Check sheet for the modelled part. Datum: model origin and axes. Units: mm. A direction names the side the tool comes from. Give positions to 0.01 mm unless a question says otherwise; leave off trailing zeros. Order: outer loops, then holes, each group sorted by start corner. A loop starts at its lowest first (then second) coordinate and runs counter-clockwise, first axis right, second up. Notation, with made-up numbers: (66.25, 82.5) -> (98.25, 82.5) arc R24 cw to (98.25, 107.5) -> close; hole circle Ø2 at (84.5, 12). An arc over 180 degrees is marked (long way). Answer in a Markdown table with one row per item. Add a question column.
(1) Go/stop test with flat-tipped pins: pin 1 (12 mm diameter, centred on y = -14.5, z = -11, fed in from +X); pin 2 (1 mm diameter, centred on y = -9.5, z = -28, fed in from +X); pin 3 (6 mm diameter, centred on x = -42, y = -17.5, fed in from +Z); pin 4 (4 mm diameter, centred on x = 17.5, z = 16, fed in from -Y). Record where each tip stops, or that it passes through.
(2) Thickness scan on L1, parallel to Z at x = -53, y = -6; L2, parallel to Z at x = -33, y = -16.5; L3, parallel to Z at x = -11, y = -12.25 (3 decimals). Record the ranges inside material, lowest first. Write a range as [from, to].
(3) Cross-section at B-B (y = -9.5). State how many separate pieces and enclosed holes the cut face has, then the cut area to 3 significant figures.
(4) Cross-section at A-A (x = 0). Record the cut outline in (y, z).
(5) Release check for a two-part mould opening along Z. For faces 6 (the face through (49.733, -9.86, 5.165)), 7 (the face through (-10.34, -9.86, 48.92)), 8 (the face through (31, 0, 36)) record: released by +Z, released by -Z, zero draft, split by the parting line, or undercut.
(6) Set-up check for faces 1 (the face through (-49.72, -9.86, 5.29)), 2 (the face through (5.832, -9.86, -54.889)), 3 (the face through (10.456, -9.86, 48.895)), 4 (the face through (-7.353, -9.86, -10.17)), 5 (the face through (45.01, -9.86, 40.43)): record each of +Z, -Z, +X, -X, +Y, -Y from which the full face is reachable in a straight line by a thin tool's end or side.
```python
from build123d import *

# Parameters (mm, degrees)
F1_R     = 50
F2_DEPTH = 20
F4_DEPTH = 20
F5_R     = 45
F5_R_2   = 16
F6_DEPTH = 8
F7_R     = 10
F8_DEPTH = 25
F9_SIZE  = 2
F10_R    = 3


with BuildPart() as f2:
    # F1 (on Front) → F2 (new body)
    with BuildSketch(Plane.XZ):
        Circle(F1_R)
        with BuildLine():
            ThreePointArc((-2.05, 12.3814377194), (0, 12.55), (2.05, 12.3814377194))
            Line((2.05, 12.3814377194), (2.05, 10.2979366865))
            ThreePointArc((2.05, 10.2979366865), (3.2446784409, 9.9860934211), (4.3944904749, 9.5361655536))
            Line((4.3944904749, 9.5361655536), (5.6191416552, 11.221753297))
            ThreePointArc((5.6191416552, 11.221753297), (7.3767049163, 10.1531632794), (8.9361113321, 8.8118337626))
            Line((8.9361113321, 8.8118337626), (7.7114601519, 7.1262460192))
            ThreePointArc((7.7114601519, 7.1262460192), (8.4946784409, 6.1717451491), (9.1604349517, 5.1319033015))
            Line((9.1604349517, 5.1319033015), (11.1419621857, 5.7757405285))
            ThreePointArc((11.1419621857, 5.7757405285), (11.9357592795, 3.8781632794), (12.4089318626, 1.8764088117))
            Line((12.4089318626, 1.8764088117), (10.4274046286, 1.2325715847))
            ThreePointArc((10.4274046286, 1.2325715847), (10.4818354452, 0.6173537882), (10.5, 0))
            ThreePointArc((10.5, 0), (10.4818354452, -0.6173537882), (10.4274046286, -1.2325715847))
            Line((10.4274046286, -1.2325715847), (12.4089318626, -1.8764088117))
            ThreePointArc((12.4089318626, -1.8764088117), (11.9357592795, -3.8781632794), (11.1419621857, -5.7757405285))
            Line((11.1419621857, -5.7757405285), (9.1604349517, -5.1319033015))
            ThreePointArc((9.1604349517, -5.1319033015), (8.4946784409, -6.1717451491), (7.7114601519, -7.1262460192))
            Line((7.7114601519, -7.1262460192), (8.9361113321, -8.8118337626))
            ThreePointArc((8.9361113321, -8.8118337626), (7.3767049163, -10.1531632794), (5.6191416552, -11.221753297))
            Line((5.6191416552, -11.221753297), (4.3944904749, -9.5361655536))
            ThreePointArc((4.3944904749, -9.5361655536), (3.2446784409, -9.9860934211), (2.05, -10.2979366865))
            Line((2.05, -10.2979366865), (2.05, -12.3814377194))
            ThreePointArc((2.05, -12.3814377194), (0, -12.55), (-2.05, -12.3814377194))
            Line((-2.05, -12.3814377194), (-2.05, -10.2979366865))
            ThreePointArc((-2.05, -10.2979366865), (-3.2446784409, -9.9860934211), (-4.3944904749, -9.5361655536))
            Line((-4.3944904749, -9.5361655536), (-5.6191416552, -11.221753297))
            ThreePointArc((-5.6191416552, -11.221753297), (-7.3767049163, -10.1531632794), (-8.9361113321, -8.8118337626))
            Line((-8.9361113321, -8.8118337626), (-7.7114601519, -7.1262460192))
            ThreePointArc((-7.7114601519, -7.1262460192), (-8.4946784409, -6.1717451491), (-9.1604349517, -5.1319033015))
            Line((-9.1604349517, -5.1319033015), (-11.1419621857, -5.7757405285))
            ThreePointArc((-11.1419621857, -5.7757405285), (-11.9357592795, -3.8781632794), (-12.4089318626, -1.8764088117))
            Line((-12.4089318626, -1.8764088117), (-10.4274046286, -1.2325715847))
            ThreePointArc((-10.4274046286, -1.2325715847), (-10.5, 0), (-10.4274046286, 1.2325715847))
            Line((-10.4274046286, 1.2325715847), (-12.4089318626, 1.8764088117))
            ThreePointArc((-12.4089318626, 1.8764088117), (-11.9357592795, 3.8781632794), (-11.1419621857, 5.7757405285))
            Line((-11.1419621857, 5.7757405285), (-9.1604349517, 5.1319033015))
            ThreePointArc((-9.1604349517, 5.1319033015), (-8.4946784409, 6.1717451491), (-7.7114601519, 7.1262460192))
            Line((-7.7114601519, 7.1262460192), (-8.9361113321, 8.8118337626))
            ThreePointArc((-8.9361113321, 8.8118337626), (-7.3767049163, 10.1531632794), (-5.6191416552, 11.221753297))
            Line((-5.6191416552, 11.221753297), (-4.3944904749, 9.5361655536))
            ThreePointArc((-4.3944904749, 9.5361655536), (-3.2446784409, 9.9860934211), (-2.05, 10.2979366865))
            Line((-2.05, 10.2979366865), (-2.05, 12.3814377194))
        make_face(mode=Mode.SUBTRACT)
    extrude(amount=F2_DEPTH)

    # F3 (on Front) → F4 (join)
    with BuildSketch(Plane.XZ):
        with BuildLine():
            ThreePointArc((6.0454455831, 49.6331803102), (5.6999328162, 54.9765582241), (5.0372687356, 60.2899321917))
            ThreePointArc((5.0372687356, 60.2899321917), (0, 60.5), (-5.0372687356, 60.2899321917))
            ThreePointArc((-5.0372687356, 60.2899321917), (-5.6999328162, 54.9765582241), (-6.0454455831, 49.6331803102))
            ThreePointArc((-6.0454455831, 49.6331803102), (0, 50), (6.0454455831, 49.6331803102))
        make_face()
        with BuildLine():
            ThreePointArc((19.9203506586, 57.1264354711), (17.1538330068, 52.5419565819), (14.6648437927, 47.8010706631))
            ThreePointArc((14.6648437927, 47.8010706631), (20.3368321538, 45.6772728821), (25.7104224964, 42.8832621783))
            ThreePointArc((25.7104224964, 42.8832621783), (27.5681284731, 47.905213503), (29.1238986033, 53.0287519196))
            ThreePointArc((29.1238986033, 53.0287519196), (24.6075669061, 55.2695001874), (19.9203506586, 57.1264354711))
        make_face()
        with BuildLine():
            ThreePointArc((41.4335604532, 44.0852590802), (37.0415452653, 41.022373318), (32.8394484508, 37.7037216393))
            ThreePointArc((32.8394484508, 37.7037216393), (37.1572412739, 33.4565303179), (40.9298337882, 28.7184384337))
            ThreePointArc((40.9298337882, 28.7184384337), (44.6695442683, 32.5506221621), (48.1747418201, 36.5984186894))
            ThreePointArc((48.1747418201, 36.5984186894), (44.9602619414, 40.4824016847), (41.4335604532, 44.0852590802))
        make_face()
        with BuildLine():
            ThreePointArc((55.7825312334, 23.4213408923), (50.5244378355, 22.4096490308), (45.3358141347, 21.0870566164))
            ThreePointArc((45.3358141347, 21.0870566164), (47.5528258148, 15.4508497187), (49.0721049822, 9.587935785))
            ThreePointArc((49.0721049822, 9.587935785), (54.0471900496, 11.5677325362), (58.8957345225, 13.8398863816))
            ThreePointArc((58.8957345225, 13.8398863816), (57.5389192359, 18.6955281597), (55.7825312334, 23.4213408923))
        make_face()
        with BuildLine():
            ThreePointArc((60.486195595, -1.2923399121), (55.2711961039, -0.077907159), (49.9932056918, 0.8242479348))
            ThreePointArc((49.9932056918, 0.8242479348), (49.9983013941, 0.4121379686), (50, 0))
            ThreePointArc((50, 0), (49.6813253191, -5.6361258444), (48.7293634187, -11.2004080646))
            ThreePointArc((48.7293634187, -11.2004080646), (54.0795856679, -11.4153231348), (59.433119675, -11.3116880129))
            ThreePointArc((59.433119675, -11.3116880129), (60.1685746698, -6.3239720277), (60.486195595, -1.2923399121))
        make_face()
        with BuildLine():
            ThreePointArc((54.7312472383, -25.7825634052), (50.4610624428, -22.5519924933), (46.0063178108, -19.5810807029))
            ThreePointArc((46.0063178108, -19.5810807029), (43.3012701892, -25), (39.9608722277, -30.0520996073))
            ThreePointArc((39.9608722277, -30.0520996073), (44.7611296266, -32.4245657308), (49.6939785027, -34.5073687866))
            ThreePointArc((49.6939785027, -34.5073687866), (52.394536929, -30.25), (54.7312472383, -25.7825634052))
        make_face()
        with BuildLine():
            ThreePointArc((39.5127690163, -45.8147474582), (36.9257526611, -41.1266334471), (34.064519626, -36.6006625985))
            ThreePointArc((34.064519626, -36.6006625985), (29.3892626146, -40.4508497187), (24.2827831954, -43.7075101131))
            ThreePointArc((24.2827831954, -43.7075101131), (27.7030676308, -47.827306344), (31.3622969917, -51.7364120075))
            ThreePointArc((31.3622969917, -51.7364120075), (35.5610077637, -48.9455281597), (39.5127690164, -45.8147474582))
        make_face()
        with BuildLine():
            ThreePointArc((17.4621740692, -57.9251454618), (17.0056447843, -52.5901058542), (16.2326565314, -47.2916574242))
            ThreePointArc((16.2326565314, -47.2916574242), (10.3955845409, -48.9073800367), (4.4059803465, -49.8054950501))
            ThreePointArc((4.4059803465, -49.8054950501), (5.8548935672, -54.9602711929), (7.6077894133, -60.0197595817))
            ThreePointArc((7.6077894133, -60.0197595817), (12.5786572945, -59.1779298444), (17.4621740692, -57.9251454618))
        make_face()
        with BuildLine():
            ThreePointArc((-4.4059803465, -49.8054950501), (-10.3955845409, -48.9073800367), (-16.2326565314, -47.2916574242))
            ThreePointArc((-16.2326565314, -47.2916574242), (-17.0056447843, -52.5901058542), (-17.4621740692, -57.9251454618))
            ThreePointArc((-17.4621740692, -57.9251454618), (-12.5786572945, -59.1779298444), (-7.6077894133, -60.0197595817))
            ThreePointArc((-7.6077894133, -60.0197595817), (-5.8548935672, -54.9602711929), (-4.4059803465, -49.8054950501))
        make_face()
        with BuildLine():
            ThreePointArc((-24.2827831954, -43.7075101131), (-29.3892626146, -40.4508497187), (-34.064519626, -36.6006625985))
            ThreePointArc((-34.064519626, -36.6006625985), (-36.9257526611, -41.1266334471), (-39.5127690164, -45.8147474582))
            ThreePointArc((-39.5127690164, -45.8147474582), (-35.5610077637, -48.9455281597), (-31.3622969917, -51.7364120075))
            ThreePointArc((-31.3622969917, -51.7364120075), (-27.7030676308, -47.827306344), (-24.2827831954, -43.7075101131))
        make_face()
        with BuildLine():
            ThreePointArc((-39.9608722277, -30.0520996073), (-43.3012701892, -25), (-46.0063178108, -19.5810807029))
            ThreePointArc((-46.0063178108, -19.5810807029), (-50.4610624428, -22.5519924933), (-54.7312472383, -25.7825634052))
            ThreePointArc((-54.7312472383, -25.7825634052), (-52.394536929, -30.25), (-49.6939785027, -34.5073687866))
            ThreePointArc((-49.6939785027, -34.5073687866), (-44.7611296266, -32.4245657308), (-39.9608722277, -30.0520996073))
        make_face()
        with BuildLine():
            ThreePointArc((-48.7293634187, -11.2004080646), (-49.7260947684, -5.2264231634), (-49.9932056918, 0.8242479348))
            ThreePointArc((-49.9932056918, 0.8242479348), (-55.2711961039, -0.077907159), (-60.486195595, -1.2923399121))
            ThreePointArc((-60.486195595, -1.2923399121), (-60.1685746698, -6.3239720277), (-59.433119675, -11.3116880129))
            ThreePointArc((-59.433119675, -11.3116880129), (-54.0795856679, -11.4153231348), (-48.7293634187, -11.2004080646))
        make_face()
        with BuildLine():
            ThreePointArc((-49.0721049822, 9.587935785), (-47.5528258148, 15.4508497187), (-45.3358141347, 21.0870566164))
            ThreePointArc((-45.3358141347, 21.0870566164), (-50.5244378355, 22.4096490308), (-55.7825312334, 23.4213408923))
            ThreePointArc((-55.7825312334, 23.4213408923), (-57.5389192359, 18.6955281597), (-58.8957345225, 13.8398863816))
            ThreePointArc((-58.8957345225, 13.8398863816), (-54.0471900496, 11.5677325362), (-49.0721049822, 9.587935785))
        make_face()
        with BuildLine():
            ThreePointArc((-40.9298337882, 28.7184384337), (-37.1572412739, 33.4565303179), (-32.8394484508, 37.7037216393))
            ThreePointArc((-32.8394484508, 37.7037216393), (-37.0415452653, 41.022373318), (-41.4335604532, 44.0852590802))
            ThreePointArc((-41.4335604532, 44.0852590802), (-44.9602619414, 40.4824016847), (-48.1747418201, 36.5984186894))
            ThreePointArc((-48.1747418201, 36.5984186894), (-44.6695442683, 32.5506221621), (-40.9298337882, 28.7184384337))
        make_face()
        with BuildLine():
            ThreePointArc((-25.7104224964, 42.8832621783), (-20.3368321538, 45.6772728821), (-14.6648437927, 47.8010706631))
            ThreePointArc((-14.6648437927, 47.8010706631), (-17.1538330068, 52.5419565819), (-19.9203506586, 57.1264354711))
            ThreePointArc((-19.9203506586, 57.1264354711), (-24.6075669061, 55.2695001874), (-29.1238986033, 53.0287519196))
            ThreePointArc((-29.1238986033, 53.0287519196), (-27.5681284731, 47.905213503), (-25.7104224964, 42.8832621783))
        make_face()
    extrude(amount=F4_DEPTH)

    # F5 (on Front) → F6 (cut)
    with BuildSketch(Plane.XZ):
        Circle(F5_R)
        Circle(F5_R_2, mode=Mode.SUBTRACT)
    extrude(amount=F6_DEPTH, mode=Mode.SUBTRACT)

    # F7 (on Front) → F8 (cut)
    with BuildSketch(Plane.XZ):
        with Locations((0, 31)):
            Circle(F7_R)
        with Locations((-24.2367759565, 19.3281838576)):
            Circle(F7_R)
        with Locations((-30.2227652776, -6.8981489526)):
            Circle(F7_R)
        with Locations((-13.4503959126, -27.930034905)):
            Circle(F7_R)
        with Locations((13.4503959126, -27.930034905)):
            Circle(F7_R)
        with Locations((30.2227652776, -6.8981489526)):
            Circle(F7_R)
        with Locations((24.2367759565, 19.3281838576)):
            Circle(F7_R)
    extrude(amount=F8_DEPTH, mode=Mode.SUBTRACT)

    # F9
    f9_edges = [f2.edges().sort_by_distance(p)[0] for p in [
        (-45, 0, 0),
        (-45, -8, 0),
    ]]
    chamfer(f9_edges, length=F9_SIZE)

    # F10
    f10_edges = [f2.edges().sort_by_distance(p)[0] for p in [
        (-16, -8, 0),
    ]]
    fillet(f10_edges, radius=F10_R)


solid = f2.part
```
Answer below:
| question | item | result |
|---|---|---|
| 1 | pin 1 | stops at x = 60.29 |
| 1 | pin 2 | stops at x = 53.89 |
| 1 | pin 3 | stops at z = 44.09 |
| 1 | pin 4 | passes through |
| 2 | L1 | z = [-29.18, -24.42], [-11.4, 0.35], [11.12, 22.93] |
| 2 | L2 | z = [-50.71, -16.5], [2.71, 14.51], [24.15, 37.84] |
| 2 | L3 | z = [-59.492, -37.625], [-18.235, -5.73], [-1.419, 1.419], [5.73, 48.775] |
| 3 | separate pieces | 1 |
| 3 | enclosed holes | 8 |
| 3 | area | 7,010 mm² |
| 4 | outline | (-20, -50) -> (0, -50) -> (0, -47) -> (-2, -45) -> (-6, -45) -> (-8, -43) -> (-8, -19) arc R3 cw to (-5, -16) -> (0, -16) -> (0, -12.55) -> (-20, -12.55) -> close; (-20, 12.55) -> (0, 12.55) -> (0, 16) -> (-5, 16) arc R3 cw to (-8, 19) -> (-8, 21) -> (-20, 21) -> close; (-20, 41) -> (-8, 41) -> (-8, 43) -> (-6, 45) -> (-2, 45) -> (0, 47) -> (0, 60.5) -> (-20, 60.5) -> close |
| 5 | face 6 | undercut |
| 5 | face 7 | released by +Z |
| 5 | face 8 | zero draft |
| 6 | face 1 | -X, +Y, -Y |
| 6 | face 2 | -Z, +Y, -Y |
| 6 | face 3 | +Z, +Y, -Y |
| 6 | face 4 | +Y, -Y |
| 6 | face 5 | +Z, +X, +Y, -Y |
